Input: part model. Units: mm. Frame: model coordinates. Face numbers are marked on the shaded views. A direction names the side the tool comes from. Round coordinates to 2 decimals unless told otherwise and drop trailing zeros. Order: outer loops, then holes, each group sorted by start corner. A loop starts at its lowest first (then second) coordinate and runs counter-clockwise, first axis right, second up. Notation, with made-up numbers: (2.25, 31) -> (23.25, 31) arc R16 ccw to (23.25, 59) -> close; hole circle Ø2 at (-5, 79). An arc over 180 degrees is marked (long way). Answer as CSV lines item,"result". Start each with the question number.
1) Access query for the marked faces 1 and 2. Directions: +Z, -Z, +X, -X, +Y, -Y. A direction counts if a zero-diameter tool reaches every point of the face in a straight line with its end or side. Return the directions, or none.
2) Section query B-B, the plane z = 32.5. Output: boundary loops of the cut face in (x, y), and give its area (3 significant figures).
3) First-contact query: P1, Ø12, axis at x = -24.5, y = 60.5, coming from the +Z side; P2, Ø2, axis at x = -36.54, z = 50.54, coming from the +Y side; P3, Ø12.5, axis at x = -15.5, z = 45.5, coming from the +Y side. Flat tips, straight axial feed; report the tip coordinate or a pass-through.
4) Section query D-D, the plane y = 51.5. Output: boundary loops of the cut face in (x, z).
5) Section query A-A, the plane x = -36.54. Output: boundary loops of the cut face in (y, z).
6) Section query C-C, the plane x = -15.5. Output: boundary loops of the cut face in (y, z).
7) Line query: L1, parallel to Y at x = -32, z = 12.3; L2, parallel to Z at x = -36.54, y = 40.2; L3, parallel to Z at x = -14, y = 56. Output: solid intervals per line, ascending.
Solid Edge part; units mm, degrees
sketch "Sketch1" plane through (0, 0, 0) normal (1, 0, 0) x (0, 1, 0)
  line L0 (37.5493, 56.0875) -> (41.0493, 56.0875)
  line L1 (41.0493, 56.0875) -> (41.0493, 14.0875)
  line L2 (41.0493, 14.0875) -> (86.0493, 14.0875)
  line L3 (86.0493, 14.0875) -> (86.0493, 10.5875)
  line L4 (86.0493, 10.5875) -> (37.5493, 10.5875)
  line L5 (37.5493, 10.5875) -> (37.5493, 56.0875)
  dimension "D1" = 37.5493
  dimension "D2" = 41.0493
  dimension "D3" = 37.5493
  dimension "D4" = 86.0493
  dimension "D5" = 41.0493
extrude "Protrusion1" add sketch "Sketch1" against normal blind 42
sketch "Sketch2" plane through (-21, 37.5493, 33.3375) normal (0, -1, 0) x (1, 0, 0)
  circle A0 centre (-15.54, -13.79) radius 1.23
  circle A1 centre (15.45, -13.79) radius 1.23
  circle A2 centre (-15.54, 17.2) radius 1.23
  circle A3 centre (15.45, 17.2) radius 1.23
  dimension "D1" = 15.54
extrude "Cutout1" cut sketch "Sketch2" against normal through all
sketch "Sketch3" plane through (-21, 37.5493, 33.3375) normal (0, -1, 0) x (1, 0, 0)
  circle A0 centre (-0.05, 1.71) radius 11.05
extrude "Cutout2" cut sketch "Sketch3" against normal through all
sketch "Sketch4" plane through (-21, 61.7993, 10.5875) normal (0, 0, -1) x (1, 0, 0)
  circle A0 centre (-11, -14.25) radius 1.5
  circle A1 centre (11, -14.25) radius 1.5
  circle A2 centre (-11, 14.25) radius 1.5
  circle A3 centre (11, 14.25) radius 1.5
  dimension "D1" = 11
extrude "Cutout3" cut sketch "Sketch4" against normal up to next
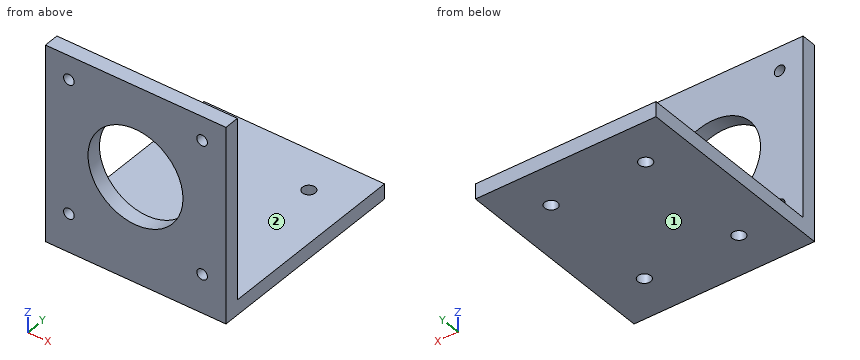
Findings:
1,face 1,"-Z, +X, -X, +Y, -Y"
1,face 2,"+Z, +X, -X, +Y"
2,outline,"(-42, 37.55) -> (-31.8, 37.55) -> (-31.8, 41.05) -> (-42, 41.05) -> close; (-10.3, 37.55) -> (0, 37.55) -> (0, 41.05) -> (-10.3, 41.05) -> close"
2,area,"71.7 mm^2"
3,P1,"stops at z = 14.09"
3,P2,"passes through"
3,P3,"stops at y = 41.05"
4,outline,"(-42, 10.59) -> (0, 10.59) -> (0, 14.09) -> (-42, 14.09) -> close"
5,outline,"(37.55, 10.59) -> (86.05, 10.59) -> (86.05, 14.09) -> (41.05, 14.09) -> (41.05, 18.32) -> (37.55, 18.32) -> close; (37.55, 20.78) -> (41.05, 20.78) -> (41.05, 49.31) -> (37.55, 49.31) -> close; (37.55, 51.77) -> (41.05, 51.77) -> (41.05, 56.09) -> (37.55, 56.09) -> close"
6,outline,"(37.55, 10.59) -> (86.05, 10.59) -> (86.05, 14.09) -> (41.05, 14.09) -> (41.05, 25.49) -> (37.55, 25.49) -> close; (37.55, 44.6) -> (41.05, 44.6) -> (41.05, 56.09) -> (37.55, 56.09) -> close"
7,L1,"y = 37.55 to 46.05, 49.05 to 74.55, 77.55 to 86.05"
7,L2,"z = 10.59 to 18.32, 20.78 to 49.31, 51.77 to 56.09"
7,L3,"z = 10.59 to 14.09"
